Could you check a few things on this model? Use its own coordinates, in mm. A direction names the side the tool comes from. Give positions to 0.01 mm unless a question says otherwise; leave off trailing zeros. Order: outer loops, then holes, each group sorted by start corner. A loop starts at its lowest first (then second) coordinate and runs counter-clockwise, first axis right, second up.
(1) On a 3-axis mill with a long thin cutter (end or side, diameter ignored), from which of +Z, -Z, +X, -X, +Y, -Y can I reach the whole of each face in a straight line? I mean faces 1 (the flat face through (22.352, 7, 1)), 2 (the flat face through (98.1, 13, 1)), 3 (the flat face through (59, 64, 3)). Say none if no direction works.
(2) Will these pins go through, and if not, where does the flat tip stop? pin 1 (1.5 mm diameter, centred on x = 113.5, z = 2, fed in from -Y); pin 2 (1.5 mm diameter, centred on y = 9, z = 1.5, fed in from +X).
(3) Imagine slicing it at A-A, the plane z = 1.55. Write out the boundary of the cut face in (x, y).
(4) Imagine slicing it at C-C, the plane x = 109.5. Write out the boundary of the cut face in (y, z).
(5) Imagine slicing it at B-B, the plane y = 19.5. Write out the boundary of the cut face in (x, z).
(6) If I drill on probe 1 along X at (y, z) = (120.65, 2.1); probe 2 along X at (y, z) = (6, 1.6); probe 3 along Y at (x, z) = (10.46, 0.75), over which ranges is the centre line in solid material (lowest first)?
(7) If we mould it in two halves opening along Y, with no side actions, what happens to faces 4 (the flat face through (109, 25.9, 1)), 5 (the flat face through (15.748, 7, 1)), 6 (the cylindrical face through (12.15, 119.95, 1.48))? For each: released by +Y, released by -Y, zero draft, split by the parting line, or undercut.
from build123d import *

# Parameters (mm, degrees)
SKETCH_R  = 1.8288
PAD_DEPTH = 3


with BuildPart() as part:
    # Sketch → Pad (new body)
    with BuildSketch(Plane.XY):
        with BuildLine():
            Line((0, 126), (0, 1))
            ThreePointArc((0, 1), (0.292893, 0.292893), (1, 0))
            Line((1, 0), (14.748, 0))
            ThreePointArc((14.748, 0), (15.455107, 0.292893), (15.748, 1))
            Line((15.748, 12.7), (15.748, 1))
            ThreePointArc((22.352, 12.7), (19.05, 16.002), (15.748, 12.7))
            Line((22.352, 12.7), (22.352, 1))
            ThreePointArc((22.352, 1), (22.644893, 0.292893), (23.352, 0))
            Line((23.352, 0), (74.748, 0))
            ThreePointArc((74.748, 0), (75.455107, 0.292893), (75.748, 1))
            Line((75.748, 12.7), (75.748, 1))
            ThreePointArc((82.352, 12.7), (79.05, 16.002), (75.748, 12.7))
            Line((82.352, 12.7), (82.352, 1))
            ThreePointArc((82.352, 1), (82.644893, 0.292893), (83.352, 0))
            Line((83.352, 0), (97.1, 0))
            ThreePointArc((97.1, 0), (97.807107, 0.292893), (98.1, 1))
            Line((98.1, 1), (98.1, 24.9))
            ThreePointArc((99.1, 25.9), (98.392893, 25.607107), (98.1, 24.9))
            Line((99.1, 25.9), (119.2001, 25.9))
            ThreePointArc((119.2001, 25.9), (119.907207, 26.192893), (120.2001, 26.9))
            Line((120.2001, 26.9), (120.2001, 126))
            ThreePointArc((120.2001, 126), (119.907207, 126.707107), (119.2001, 127))
            Line((119.2001, 127), (1, 127))
            ThreePointArc((1, 127), (0.292893, 126.707107), (0, 126))
        make_face()
        with Locations((10.46, 120.65)):
            Circle(SKETCH_R, mode=Mode.SUBTRACT)
    extrude(amount=PAD_DEPTH)


solid = part.part
Answer block:
1. face 1: +Z, -Z, -Y
1. face 2: +Z, -Z, +X, -Y
1. face 3: +Z, +X, -X, +Y, -Y
2. pin 1: stops at y = 25.9
2. pin 2: stops at x = 98.1
3. outline: (0, 1) arc R1 ccw to (1, 0) - (14.75, 0) arc R1 ccw to (15.75, 1) - (15.75, 12.7) arc R3.3 cw to (22.35, 12.7) - (22.35, 1) arc R1 ccw to (23.35, 0) - (74.75, 0) arc R1 ccw to (75.75, 1) - (75.75, 12.7) arc R3.3 cw to (82.35, 12.7) - (82.35, 1) arc R1 ccw to (83.35, 0) - (97.1, 0) arc R1 ccw to (98.1, 1) - (98.1, 24.9) arc R1 cw to (99.1, 25.9) - (119.2, 25.9) arc R1 ccw to (120.2, 26.9) - (120.2, 126) arc R1 ccw to (119.2, 127) - (1, 127) arc R1 ccw to (0, 126) - close; hole circle Ø3.66 at (10.46, 120.65)
4. outline: (25.9, 0) - (127, 0) - (127, 3) - (25.9, 3) - close
5. outline: (0, 0) - (98.1, 0) - (98.1, 3) - (0, 3) - close
6. probe 1: x = 0 to 8.63, 12.29 to 120.2
6. probe 2: x = 0 to 15.75, 22.35 to 75.75, 82.35 to 98.1
6. probe 3: y = 0 to 118.82, 122.48 to 127
7. face 4: released by -Y
7. face 5: zero draft
7. face 6: undercut
